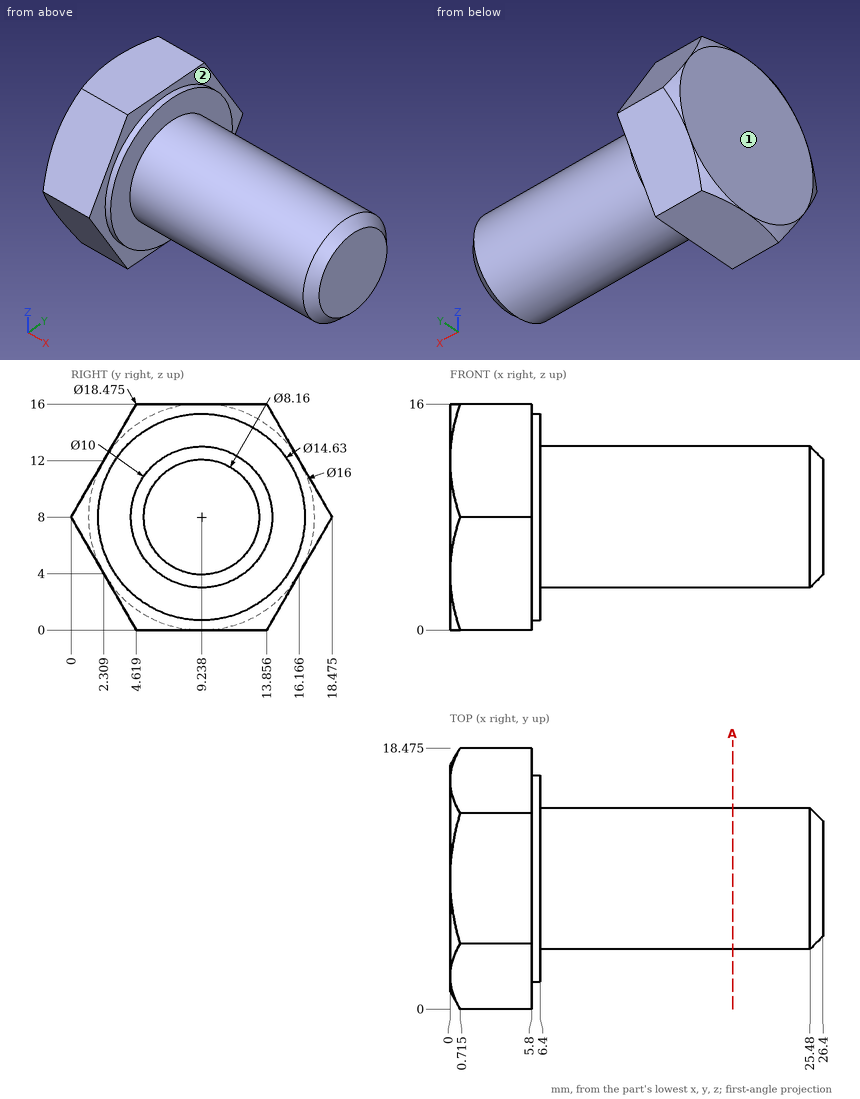
Print and shaded views of the part. All mm, measured from the part's lowest x, y and z. A direction names the side the tool comes from. Round coordinates to 2 decimals unless told otherwise and drop trailing zeros. Loops run counter-clockwise (first coordinate to the right, second up) from the corner with the lowest first, then second, coordinate; pieces in that order, holes last. Notation, with made-up numbers: (50.25, 26) -> (68.25, 26) arc R9 cw to (68.25, 36) -> close; hole circle Ø8 at (54, -17.75). An arc over 180 degrees is marked (long way). Use CSV: the item, a comma, the result in double quotes. Start each with the question number.
1) Cut at A-A, the plane x = 20. Write the cut outline in (y, z).
2) Wall check: L1, parallel to X at y = 4.5, z = 11.5; L2, parallel to Z at x = 9, y = 11.75 (1 decimal); L3, parallel to Y at x = 7.5, z = 12.5 (1 decimal). Give the ranges that are in metal, low to high. Write a range as [from, to].
3) Which spindle directions (+Z, -Z, +X, -X, +Y, -Y) get a long thin tool onto all of the face, cutting with end or side? Do the marked faces 1 and 2. Say none if no direction does.
4) Drop flat-ended pins along their axis: P1, Ø2, axis at x = 17.5, y = 2, coming from the +Z side; P2, Ø8, axis at x = 18, y = 3.5, coming from the +Z side; P3, Ø5, axis at x = 20.5, z = 11, coming from the +Y side; P4, Ø2, axis at x = 19.5, y = 11, coming from the -Z side. Give the stop position or say it passes through.
Determined:
1,outline,"circle Ø10 at (9.24, 8)"
2,L1,"x = [0, 6.4]"
2,L2,"z = [3.7, 12.3]"
2,L3,"y = [7.1, 11.4]"
3,face 1,"+Z, -Z, -X, +Y, -Y"
3,face 2,"+X"
4,P1,"passes through"
4,P2,"stops at z = 12.69"
4,P3,"stops at y = 14.21"
4,P4,"stops at z = 3.06"
